Autodesk Inventor part; units mm, degrees
ref_plane "YZ Plane" through (0, 0, 0) normal (1, 0, 0) x (0, 1, 0)
ref_plane "XZ Plane" through (0, 0, 0) normal (0, 1, 0) x (-1, 0, 0)
ref_plane "XY Plane" through (0, 0, 0) normal (0, 0, 1) x (1, 0, 0)
sketch "Skizze1" plane through (0, 0, 0) normal (1, 0, 0) x (0, 1, 0)
  line L0 (0, 0) -> (5, 0)
  line L1 (0, 5.6) -> (0, 13)
  line L2 (0, 13) -> (1, 13)
  line L3 (1, 13) -> (1, 5.6)
  line L4 (0, 5.6) -> (1, 5.6)
  dimension "d0" = 1
  dimension "d1" = 26
  dimension "d55" = 11.2
revolve "Umdrehung1" add sketch "Skizze1" angle 360 about axis through (0, 0, 0) along (0, 1, 0)
sketch "Skizze7" plane through (0, 0, 0) normal (0, 1, 0) x (-1, 0, 0)
  circle A0 centre (0, 0) radius 5.6
  line L0 (0, 0) -> (0, 5.6) construction
  line L1 (0, 0) -> (3.599611, 4.289849) construction
  arc A1 (-0.769545, 5.014619) -> (-1.915313, 5.262279) centre (-1.539091, 4.228617) ccw
  arc A2 (1.915313, 5.262279) -> (0.769545, 5.014619) centre (1.539091, 4.228617) ccw
  arc A3 (-0.769545, 5.014619) -> (0.769545, 5.014619) centre (0, 5.800622) ccw
  line L2 (1.915313, 5.262279) -> (0, 0) construction
  point P0 (0, 0)
  point P1 (0, 4.700622)
  dimension "d75" = 40
  dimension "d76" = 1.1
  dimension "d85" = 1.1
  dimension "d86" = 4.70062
  dimension "d87" = 20
sketch "Skizze7 outline for Extrusion2" plane through (0, 0, 0) normal (0, 1, 0) x (-1, 0, 0)
  arc A0 (-0.769545, 5.014619) -> (0.769545, 5.014619) centre (0, 5.800622) ccw
  arc A1 (-1.915313, 5.262279) -> (-0.769545, 5.014619) centre (-1.539091, 4.228617) cw
  arc A2 (1.915313, 5.262279) -> (-1.915313, 5.262279) centre (0, 0) ccw
  arc A3 (0.769545, 5.014619) -> (1.915313, 5.262279) centre (1.539091, 4.228617) cw
extrude "Extrusion2" add sketch "Skizze7 outline for Extrusion2" along normal up to surface (1 mm away)
pattern_circular "Runde Anordnung1" count 9 over 360 about axis through (0, -10, 0) along (0, 1, 0) of "Extrusion2"
properties part number "Encoder Disk Halter" material "Aluminium 6061"
Work out the finished part from the listing and answer in its coordinate system (mm). Give positions to 0.01 mm unless a question says otherwise; leave off trailing zeros. Write each loop counter-clockwise with the first axis right and the second up, starting at its lowest first coordinate (ties: lowest second). Pieces come first, ordered by that corner, then holes. Notation, with made-up numbers: (2.5, 37.5) - (6.5, 37.5) arc R4 cw to (6.5, 44.5) - close; hole circle Ø10 at (55.5, 80). An arc over 180 degrees is marked (long way). One line per item, written item: value. Start each with the question number.
1. Find section D-D (x = 10.25). Write down the section's boundary in (y, z), then the cut area to 3 significant figures.
2. Find section C-C (z = -3.75). Write down the section's boundary in (x, y).
3. Find section A-A (x = 0). Write down the section's boundary in (y, z).
4. Consider probe 1 along X at (y, z) = (0.75, 1); probe 2 along X at (y, z) = (0.7, -4.75); probe 3 along Z at (x, y) = (12, 0.3). Determine where each line is inside the solid, lowest interval first.
5. Find section B-B (y = 0.85). Write down the section's boundary in (x, z).
Geometry results:
1. outline: (0, -8) - (1, -8) - (1, 8) - (0, 8) - close
1. area: 16.0 mm2
2. outline: (-12.45, 0) - (-3.95, 0) - (-3.95, 1) - (-12.45, 1) - close; (3.95, 0) - (12.45, 0) - (12.45, 1) - (3.95, 1) - close
3. outline: (0, -13) - (1, -13) - (1, -5.6) - (0, -5.6) - close; (0, 4.7) - (1, 4.7) - (1, 13) - (0, 13) - close
4. probe 1: -12.96 to -4.61, 4.61 to 12.96
4. probe 2: -12.1 to -1.14, 1.14 to 12.1
4. probe 3: -5 to 5
5. outline: circle Ø26 at (0, 0); hole (-5.07, 0.11) arc R1.1 ccw to (-4.73, -1.84) arc R1.1 cw to (-3.96, -3.17) arc R1.1 ccw to (-3.6, -4.29) arc R1.1 ccw to (-2.44, -4.45) arc R1.1 cw to (-0.99, -4.98) arc R1.1 ccw to (0.99, -4.98) arc R1.1 cw to (2.44, -4.45) arc R1.1 ccw to (3.6, -4.29) arc R1.1 ccw to (3.96, -3.17) arc R1.1 cw to (4.73, -1.84) arc R1.1 ccw to (5.07, 0.11) arc R1.1 cw to (4.8, 1.63) arc R1.1 ccw to (3.81, 3.35) arc R1.1 cw to (2.63, 4.34) arc R1.1 ccw to (0.77, 5.01) arc R1.1 cw to (-0.77, 5.01) arc R1.1 ccw to (-2.63, 4.34) arc R1.1 cw to (-3.81, 3.35) arc R1.1 ccw to (-4.8, 1.63) arc R1.1 cw to start
